Source: CAD feature listing. Evaluate the final solid. Frame: model axes, mm. Round coordinates to 2 decimals unless told otherwise and drop trailing zeros. Order: outer loops, then holes, each group sorted by start corner. A loop starts at its lowest first (then second) coordinate and runs counter-clockwise, first axis right, second up. Notation, with made-up numbers: (-36.5, 22.5) - (-27.5, 22.5) arc R14 cw to (-27.5, 36.5) - close; hole circle Ø3 at (-1.75, 14). An arc over 180 degrees is marked (long way). Use one line per item in the form item = value. Start each with the question number.
Q1. Pin query (flat end, axial travel): pin 1 Ø0.9 at (y, z) = (2, 0) entering from +X; pin 2 Ø1.5 at (x, y) = (33, 2.5) entering from +Z; pin 3 Ø2.5 at (y, z) = (2.54, -50.8) entering from -X. Return the tip coordinate at first contact, or that it passes through.
Q2. Cut plane B-B, the plane x = 81. Return the cut outline in (y, z), and give its area (3 significant figures).
Q3. Ray query, line 1 (X direction, y = 1.75, z = 68.58) (1 decimal); line 2 (X direction, y = 1.4, z = -44.45); line 3 (Y direction, x = -181, z = 0). Return the intervals inside material, ascending. Write a range as [from, to].
Q4. Cut plane A-A, the plane z = 68.58. Return the cut outline in (x, y) (1 decimal).
Q5. Draft query along Z for faces 1 (the cylindrical face through (123.056, 2.502, -41.405)), 2 (the flat face through (-3, 5.075, -5)). Return one class per face: released by +Z, released by -Z, zero draft, split by the parting line, or undercut.
from build123d import *

# Parameters (mm, degrees)
SKETCH1_R               = 22.225
SKETCH1_W               = 373.38
SKETCH1_H               = 127
BOSS_EXTRUDE1_DEPTH     = 5.07492
SKETCH1_5_R             = 6.2865
CUT_EXTRUDE1_DEPTH      = 208.664293845
CUT_EXTRUDE2_DEPTH      = 208.664293845
CUT_EXTRUDE2_DEPTH_BACK = 208.664293845
SKETCH1_7_R             = 3.048
SKETCH1_8_R             = 2.54
SKETCH1_8_R_2           = 3.175
CUT_EXTRUDE3_DEPTH      = 208.664293845
SKETCH2_R               = 1.4224
CUT_EXTRUDE4_DEPTH      = 12.7
CUT_EXTRUDE5_START      = -12.7
SKETCH3_R               = 1.4224
CUT_EXTRUDE5_DEPTH      = 12.7


with BuildPart() as part:
    # Sketch1 → Boss-Extrude1 (new body)
    with BuildSketch(Plane(origin=(0, 0, 0), x_dir=(1, 0, 0), z_dir=(0, 1, 0))):
        with Locations((-123.19, -68.58)):
            Circle(SKETCH1_R)
        with Locations((123.19, -68.58)):
            Circle(SKETCH1_R)
        Rectangle(SKETCH1_W, SKETCH1_H)
    extrude(amount=BOSS_EXTRUDE1_DEPTH)

    # Sketch1_5 → Cut-Extrude1 (cut, through all)
    with BuildSketch(Plane(origin=(0, 0, 0), x_dir=(1, 0, 0), z_dir=(0, 1, 0))):
        with Locations(Location((-123.19, -68.58, 0), (0, 0, 90))):
            Circle(SKETCH1_5_R)
        with Locations(Location((123.19, -68.58, 0), (0, 0, 90))):
            Circle(SKETCH1_5_R)
    extrude(amount=CUT_EXTRUDE1_DEPTH, mode=Mode.SUBTRACT)

    # Sketch1_7 → Cut-Extrude2 (cut, two sides: drawn at the far end of the back side and taken through both)
    with BuildSketch(Plane(origin=(0, 0, 0), x_dir=(1, 0, 0), z_dir=(0, 1, 0)).offset(-CUT_EXTRUDE2_DEPTH_BACK)):
        with Locations(Location((-123.19, 44.45, 0), (0, 0, 90))):
            Circle(SKETCH1_7_R)
        with Locations(Location((123.19, 44.45, 0), (0, 0, 90))):
            Circle(SKETCH1_7_R)
    extrude(amount=CUT_EXTRUDE2_DEPTH + CUT_EXTRUDE2_DEPTH_BACK, mode=Mode.SUBTRACT)

    # Sketch1_8 → Cut-Extrude3 (cut, through all)
    with BuildSketch(Plane(origin=(0, 0, 0), x_dir=(1, 0, 0), z_dir=(0, 1, 0))):
        with Locations(Location((-33.02, -37.338, 0), (0, 0, 90))):
            Circle(SKETCH1_8_R)
        with Locations(Location((17.78, -37.338, 0), (0, 0, 90))):
            Circle(SKETCH1_8_R)
        with Locations(Location((0, -54.864, 0), (0, 0, 90))):
            Circle(SKETCH1_8_R_2)
    extrude(amount=CUT_EXTRUDE3_DEPTH, mode=Mode.SUBTRACT)

    # Sketch2 → Cut-Extrude4 (cut)
    with BuildSketch(Plane(origin=(186.69, 0, 0), x_dir=(0, 0, -1), z_dir=(1, 0, 0))):
        with Locations((0, 2.53746)):
            Circle(SKETCH2_R)
        with Locations((-50.8, 2.53746)):
            Circle(SKETCH2_R)
        with Locations((50.8, 2.53746)):
            Circle(SKETCH2_R)
    extrude(amount=-CUT_EXTRUDE4_DEPTH, mode=Mode.SUBTRACT)

    # Sketch3 → Cut-Extrude5 (cut)
    with BuildSketch(Plane.ZY.offset(186.69).offset(CUT_EXTRUDE5_START)):
        with Locations(Location((-50.8, 2.53746, 0), (0, 0, 180))):
            Circle(SKETCH3_R)
        with Locations(Location((0, 2.53746, 0), (0, 0, 180))):
            Circle(SKETCH3_R)
    extrude(amount=CUT_EXTRUDE5_DEPTH, mode=Mode.SUBTRACT)


solid = part.part
Completed:
q1.pin_1 = 173.99
q1.pin_2 = 63.5
q1.pin_3 = -173.99
q2.outline = (0, -63.5) - (5.07, -63.5) - (5.07, 63.5) - (0, 63.5) - close
q2.area = 645 mm2
q3.line_1 = [-145.4, -129.5], [-116.9, -101], [101, 116.9], [129.5, 145.4]
q3.line_2 = [-186.69, -126.24], [-120.14, 120.14], [126.24, 186.69]
q3.line_3 = [0, 1.12], [3.96, 5.07]
q4.outline = (-145.4, 0) - (-129.5, 0) - (-129.5, 5.1) - (-145.4, 5.1) - close; (-116.9, 0) - (-101, 0) - (-101, 5.1) - (-116.9, 5.1) - close; (101, 0) - (116.9, 0) - (116.9, 5.1) - (101, 5.1) - close; (129.5, 0) - (145.4, 0) - (145.4, 5.1) - (129.5, 5.1) - close
q5.face_1 = undercut
q5.face_2 = zero draft
